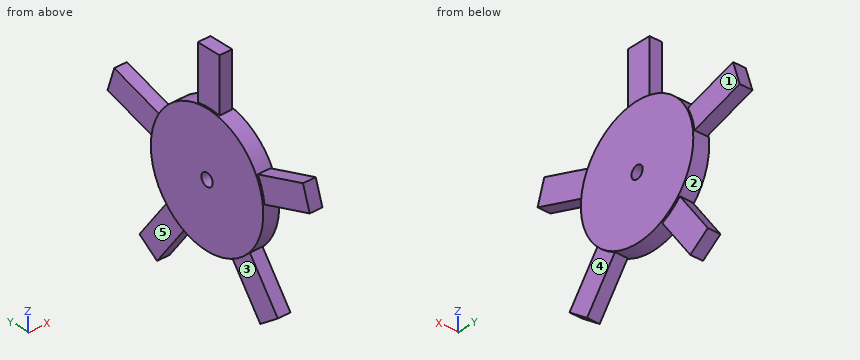
from build123d import *

# Parameters (mm, degrees)
F2_R     = 25.4
F2_R_2   = 2.54
F3_DEPTH = 3.175
F4_W     = 9.7803566605
F4_H     = 21.473386322
F5_DEPTH = 2.54


# Not quite as in the source:
# - the program builds the solid bodies; features that only make, move or delete a surface that nothing else refers to are left out


with BuildPart() as f3:
    # F2 (on Right) → F3 (new body, symmetric)
    with BuildSketch(Plane.YZ):
        Circle(F2_R)
        Circle(F2_R_2, mode=Mode.SUBTRACT)
    extrude(amount=F3_DEPTH, both=True)

    # F4 (on Right) → F5 (join, symmetric)
    with BuildSketch(Plane.YZ):
        with Locations((0, 35.6615032084)):
            Rectangle(F4_W, F4_H)
        Polygon((-45.638455211, 9.6869952197), (-25.2160512226, 3.0513539194), (-22.1937548034, 12.353025853), (-42.6161587919, 18.9886671533), align=None)
        Polygon((-23.3159381842, -40.4113040748), (-10.6941983874, -23.0389696135), (-18.6066731367, -17.2902202063), (-31.2284129336, -34.6625546676), align=None)
        Polygon((31.2284129336, -34.6625546676), (18.6066731367, -17.2902202063), (10.6941983874, -23.0389696135), (23.3159381842, -40.4113040748), align=None)
        Polygon((42.6161587919, 18.9886671533), (22.1937548034, 12.353025853), (25.2160512226, 3.0513539194), (45.638455211, 9.6869952197), align=None)
    extrude(amount=F5_DEPTH, both=True)


solid = f3.part
Design review of the part built by this model. Coordinates are the model's own, in mm. Face numbers are marked on the shaded views. A direction names the side the tool comes from. Coordinates: 2 decimals unless noted, no trailing zeros. Write each loop counter-clockwise with the first axis right and the second up, starting at its lowest first coordinate (ties: lowest second). Pieces come first, ordered by that corner, then holes. Notation, with made-up numbers: (39, 22.25) - (85, 22.25) arc R15 ccw to (85, 37.25) - close; hole circle Ø9 at (-21.75, 74.25). An arc over 180 degrees is marked (long way). One line per item, written item: value.
1) Add section B-B (z = 0). State the section outline as (x, y) points (3 decimals), plus the area to 3 significant figures.
Answer sheet:
outline: (-3.175, -25.4) - (3.175, -25.4) - (3.175, -2.54) - (-3.175, -2.54) - close; (-3.175, 2.54) - (3.175, 2.54) - (3.175, 25.4) - (-3.175, 25.4) - close
area: 290 mm2
2) Add section D-D (z = 33.5). State the section outline as (x, y) points, plus the area to 3 significant figures.
Answer sheet:
outline: (-2.54, -4.89) - (2.54, -4.89) - (2.54, 4.89) - (-2.54, 4.89) - close
area: 49.7 mm2
3) For the marked faces 3, 4 and 5, list the 3-axis set-ups (+Z, -Z, +X, -X, +Y, -Y) from which the entire face can be reached by the end or side of a thin tool; tool diameter is ignored.
Answer sheet:
face 3: -Z, -X, -Y
face 4: -Z, +X, -Y
face 5: -Z, -X, +Y
4) Add section A-A (y = 0). State the section outline as (x, z) points (3 decimals).
Answer sheet:
outline: (-3.175, -25.4) - (3.175, -25.4) - (3.175, -2.54) - (-3.175, -2.54) - close; (-3.175, 2.54) - (3.175, 2.54) - (3.175, 25.4) - (2.54, 25.4) - (2.54, 46.398) - (-2.54, 46.398) - (-2.54, 25.4) - (-3.175, 25.4) - close
5) To check wall thickness, follow probe 1 along Z at (x, y) = (-0.75, 0); probe 2 along Y at (x, z) = (1.5, -23.5); probe 3 along Y at (x, z) = (-2.5, 42). State the ranges of each line that lie inside material, in increasing order.
Answer sheet:
probe 1: z = -25.4 to -2.54, 2.54 to 46.4
probe 2: y = -23.12 to -11.03, -9.64 to 9.64, 11.03 to 23.12
probe 3: y = -4.89 to 4.89
6) Insertion check: pin 1 (8 mm diameter, centred on y = 30.5, z = 12.5, fed in from -X); pin 2 (6 mm diameter, centred on y = 19.5, z = -29, fed in from +X); pin 3 (6 mm diameter, centred on y = 0, z = 0, fed in from +X) (3 decimals). Each pin has a flat end and moves straight along its axis. Give the tip position at first contact, or say it passes through.
Answer sheet:
pin 1: stops at x = -2.54
pin 2: stops at x = 2.54
pin 3: stops at x = 3.175
7) Add section C-C (x = 1.25). State the section outline as (y, z) points, plus the area to 3 significant figures.
Answer sheet:
outline: (-45.64, 9.69) - (-25.22, 3.05) arc R25.4 ccw to (-18.61, -17.29) - (-31.23, -34.66) - (-23.32, -40.41) - (-10.69, -23.04) arc R25.4 ccw to (10.69, -23.04) - (23.32, -40.41) - (31.23, -34.66) - (18.61, -17.29) arc R25.4 ccw to (25.22, 3.05) - (45.64, 9.69) - (42.62, 18.99) - (22.19, 12.35) arc R25.4 ccw to (4.89, 24.92) - (4.89, 46.4) - (-4.89, 46.4) - (-4.89, 24.92) arc R25.4 ccw to (-22.19, 12.35) - (-42.62, 18.99) - close; hole circle Ø5.08 at (0, 0)
area: 3,040 mm2
8) Mouldability with a two-part tool opening along Z and no side actions: class the marked faces 1 and 2 as +Z half, -Z half, draft (parallel to the pull), parting line (faces both ways), or undercut.
Answer sheet:
face 1: draft
face 2: undercut
